Autodesk Inventor part; units mm, degrees
ref_plane "YZ Plane" through (0, 0, 0) normal (1, 0, 0) x (0, 1, 0)
ref_plane "XZ Plane" through (0, 0, 0) normal (0, 1, 0) x (-1, 0, 0)
ref_plane "XY Plane" through (0, 0, 0) normal (0, 0, 1) x (1, 0, 0)
sketch "Sketch1" plane through (0, 0, 0) normal (0, 1, 0) x (-1, 0, 0)
  line L0 (24.9723, 27.098) -> (-43.9316, 27.098)
  line L1 (-43.9316, 27.098) -> (-43.9316, -17.4091)
  line L2 (-43.9316, -17.4091) -> (24.9723, -17.4091)
  line L3 (24.9723, -17.4091) -> (24.9723, 27.098)
  circle A0 centre (9.5704, -1.5056) radius 3.81
  circle A1 centre (-3.1296, -1.5056) radius 3.81
  circle A2 centre (-15.8296, -1.5056) radius 3.81
  circle A3 centre (-28.5296, -1.5056) radius 3.81
  circle A4 centre (9.5704, 11.1944) radius 3.81
  circle A5 centre (-3.1296, 11.1944) radius 3.81
  circle A6 centre (-15.8296, 11.1944) radius 3.81
  circle A7 centre (-28.5296, 11.1944) radius 3.81
  line L4 (24.9723, -17.4091) -> (23.4483, -17.4091)
  line L5 (23.4483, -17.4091) -> (23.4483, 27.098)
  line L6 (-43.9316, -17.4091) -> (-42.4076, -17.4091)
  line L7 (-42.4076, -17.4091) -> (-42.4076, 27.098)
  point P0 (0, 0)
  dimension "d3" = 12.7
  dimension "d6" = 12.7
  dimension "d9" = 1.524
  dimension "d10" = 1.524
extrude "Extrusion1" add sketch "Sketch1" against normal blind 1.905 contours L5 L2 L7 L0 | A0 | A1 | A2 | A3 | A4 | A5 | A6 | A7
extrude "Extrusion2" add sketch "Sketch1" along normal blind 2.54 contours A0 | A1 | A2 | A3 | A4 | A5 | A6 | A7
chamfer "Chamfer1" distance 3.556 distance2 2.54 1 edges at (-5.7604, 2.54, 11.1944) measured on face at (-7.8424, 2.54, 10.6775)
chamfer "Chamfer2" distance 3.556 distance2 2.54 1 edges at (-5.7604, 2.54, -1.5056) measured on face at (-9.9176, 2.54, -0.5901)
chamfer "Chamfer3" distance 3.556 distance2 2.54 1 edges at (6.9396, 2.54, -1.5056) measured on face at (2.4763, 2.54, -0.5901)
chamfer "Chamfer4" distance 3.556 distance2 2.54 1 edges at (19.6396, 2.54, -1.5056) measured on face at (16.7802, 2.54, -2.3477)
chamfer "Chamfer5" distance 3.556 distance2 2.54 1 edges at (32.3396, 2.54, -1.5056) measured on face at (28.1824, 2.54, -0.5901)
chamfer "Chamfer6" distance 3.556 distance2 2.54 1 edges at (6.9396, 2.54, 11.1944) measured on face at (2.382, 2.54, 9.9337)
chamfer "Chamfer7" distance 3.556 distance2 2.54 1 edges at (19.6396, 2.54, 11.1944) measured on face at (16.7802, 2.54, 10.3523)
chamfer "Chamfer8" distance 3.556 distance2 2.54 1 edges at (32.3396, 2.54, 11.1944) measured on face at (28.1824, 2.54, 12.1099)
sketch "Sketch2" plane through (42.4076, 0, 27.098) normal (1, 0, 0) x (0, 0, -1)
  line L0 (19.1798, 6.2965) -> (19.1798, 7.6808)
  arc A0 (21.1991, 9.7001) -> (19.1798, 7.6808) centre (21.1991, 7.6808) ccw
  line L1 (21.1991, 9.7001) -> (26.1711, 9.7001)
  arc A1 (27.8729, 7.9983) -> (26.1711, 9.7001) centre (26.1711, 7.9983) ccw
  line L2 (27.8729, 7.9983) -> (27.8729, 6.2965)
  arc A2 (27.2379, 5.6615) -> (27.8729, 6.2965) centre (27.2379, 6.2965) ccw
  line L3 (27.2379, 5.6615) -> (19.8148, 5.6615)
  arc A3 (19.1798, 6.2965) -> (19.8148, 5.6615) centre (19.8148, 6.2965) ccw
  line L4 (26.8541, 21.209) -> (26.8541, 19.8247)
  arc A4 (24.8348, 17.8054) -> (26.8541, 19.8247) centre (24.8348, 19.8247) ccw
  line L5 (24.8348, 17.8054) -> (19.8628, 17.8054)
  arc A5 (18.161, 19.5072) -> (19.8628, 17.8054) centre (19.8628, 19.5072) ccw
  line L6 (18.161, 19.5072) -> (18.161, 21.209)
  arc A6 (18.796, 21.844) -> (18.161, 21.209) centre (18.796, 21.209) ccw
  line L7 (18.796, 21.844) -> (26.2191, 21.844)
  arc A7 (26.8541, 21.209) -> (26.2191, 21.844) centre (26.2191, 21.209) ccw
  line L8 (44.5071, 3.302) -> (0, 3.302)
  line L9 (44.5071, 3.302) -> (47.4281, 6.7381)
  line L10 (47.4281, 6.7381) -> (47.4281, 7.7839)
  line L11 (44.5071, 7.7839) -> (44.5071, 27.94)
  line L12 (42.6021, 27.94) -> (44.5071, 27.94)
  line L13 (42.6021, 26.9875) -> (42.6021, 27.94)
  line L14 (42.6021, 26.9875) -> (43.5546, 26.9875)
  line L15 (43.5546, 26.035) -> (43.5546, 26.9875)
  line L16 (0.9525, 26.035) -> (43.5546, 26.035)
  line L17 (0.9525, 26.035) -> (0.9525, 26.9875)
  line L18 (0.9525, 26.9875) -> (1.905, 26.9875)
  line L19 (1.905, 26.9875) -> (1.905, 27.94)
  line L20 (0, 27.94) -> (1.905, 27.94)
  line L21 (0, 7.7839) -> (0, 27.94)
  line L22 (0, 7.7839) -> (-2.921, 7.7839)
  line L23 (-2.921, 7.7839) -> (-2.921, 6.7381)
  line L24 (-2.921, 6.7381) -> (0, 3.302)
  line L25 (0, 0) -> (44.5071, 0)
  line L26 (0, -1.905) -> (-5.2131, 4.2274)
  line L27 (0, 3.302) -> (2.807, 0)
  line L28 (2.807, 0) -> (2.241, 0)
  line L29 (2.241, 0) -> (-3.429, 6.6699)
  line L30 (-2.921, 6.7381) -> (-3.429, 6.7381)
  line L31 (-3.429, 6.7381) -> (-3.429, 6.6699)
  line L32 (-3.429, 6.7381) -> (-3.429, 7.7839)
  line L33 (-3.429, 7.7839) -> (-3.429, 8.2919)
  line L34 (-2.921, 7.7839) -> (-1.651, 7.7839)
  line L35 (-1.651, 7.7839) -> (0, 5.8417)
  line L36 (-5.969, 8.2919) -> (-5.969, 5.6615)
  line L37 (-5.8869, 5.0201) -> (-5.969, 5.1167)
  line L38 (-5.969, 5.6615) -> (-5.969, 6.2838)
  line L39 (0, 6.2616) -> (-2.286, 8.9508)
  line L40 (-2.286, 8.9508) -> (-3.429, 7.9791)
  line L41 (-0.1085, 6.3892) -> (-0.1085, 8.8286)
  line L42 (-1.3785, 10.0986) -> (-2.794, 10.0986)
  line L43 (-5.969, 6.9236) -> (-5.969, 8.2919)
  arc A8 (-2.794, 10.0986) -> (-5.969, 6.9236) centre (-2.794, 6.9236) ccw
  line L44 (47.4281, 7.7839) -> (47.4281, 6.7381)
  line L45 (47.4281, 6.7381) -> (47.9361, 6.7381)
  line L46 (47.9361, 6.7381) -> (47.9361, 6.6699)
  line L47 (47.9361, 6.7381) -> (47.9361, 7.7839)
  line L48 (47.9361, 7.7839) -> (47.9361, 8.2919)
  line L49 (46.7931, 8.9508) -> (47.9361, 7.9791)
  arc A9 (50.4761, 6.9236) -> (47.3011, 10.0986) centre (47.3011, 6.9236) ccw
  line L50 (50.4761, 6.9236) -> (50.4761, 8.2919)
  line L51 (50.4761, 8.2919) -> (50.4761, 6.2838)
  line L52 (50.4761, 5.6615) -> (50.4761, 5.1167)
  line L53 (50.394, 5.0201) -> (50.4761, 5.1167)
  line L54 (47.4281, 6.7381) -> (44.5071, 3.302)
  line L55 (41.7002, 0) -> (42.2662, 0)
  line L56 (44.6156, 6.3892) -> (44.6156, 8.8286)
  line L57 (44.5071, 3.302) -> (41.7002, 0)
  line L58 (44.5071, 6.2616) -> (46.7931, 8.9508)
  line L59 (45.8856, 10.0986) -> (47.3011, 10.0986)
  line L60 (42.2662, 0) -> (47.9361, 6.6699)
  line L61 (44.5071, -1.905) -> (49.7202, 4.2274)
  line L62 (44.5071, 0) -> (44.5071, -1.905)
  line L63 (0, 0) -> (0, -1.905)
  line L64 (0, -1.905) -> (0, 0)
  line L65 (0, 0) -> (2.241, 0)
  line L66 (44.5071, -1.905) -> (44.5071, 0)
  line L67 (44.5071, 0) -> (42.2662, 0)
  arc A10 (-5.969, 6.2838) -> (-5.2131, 4.2274) centre (-2.794, 6.2838) ccw
  arc A11 (49.7202, 4.2274) -> (50.4761, 6.2838) centre (47.3011, 6.2838) ccw
  arc A12 (-0.1085, 8.8286) -> (-1.3785, 10.0986) centre (-1.3785, 8.8286) ccw
  arc A13 (45.8856, 10.0986) -> (44.6156, 8.8286) centre (45.8856, 8.8286) ccw
  point P0 (27.098, 0)
  point P1 (2.3019, 5.207)
  point P2 (-0.1085, 10.0986)
  point P3 (58.983, -0.9263)
  point P4 (58.983, -2.8313)
  point P5 (42.2053, 5.207)
  point P6 (44.6156, 10.0986)
  point P7 (50.4761, 6.9236)
  point P8 (-1.2941, 7.7839)
  point P9 (-0.1085, 7.7839)
  dimension "d41" = 3.302
  dimension "d42" = 0.508
  dimension "d43" = 0.508
  dimension "d44" = 1.27
  dimension "d45" = 2.54
  dimension "d46" = 3.175
  dimension "d53" = 3.175
  dimension "d56" = 1.27
extrude "Extrusion3" add sketch "Sketch2" against normal up to surface (65.8559 mm away) contours L47 L48 L49 L58 L56 A13 L59 A9 L51 A11 L61 L62 L25 L60 L46 | L31 L29 L25 L63 L26 A10 L36 A8 L42 A12 L41 L22 L39 L40 L33 L32 | L22 L41 L39
properties part number "ControllerClamp"
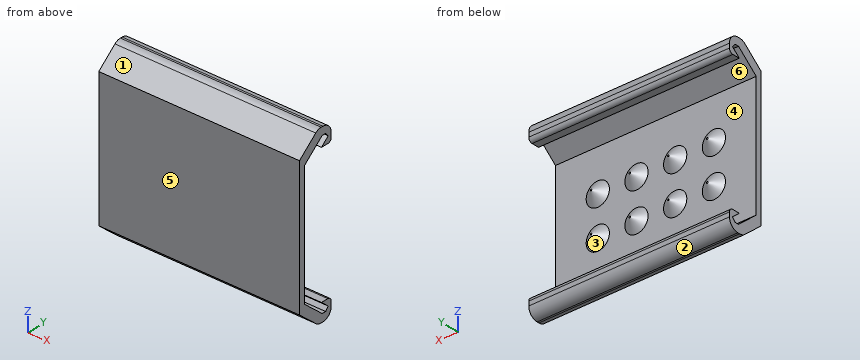
Could you check a few things on this model? Use its own coordinates, in mm. Face numbers are marked on the shaded views. A direction names the side the tool comes from. Round coordinates to 2 decimals unless told otherwise and drop trailing zeros. Order: outer loops, then holes, each group sorted by start corner. A loop starts at its lowest first (then second) coordinate and runs counter-clockwise, first axis right, second up.
(1) Please list where these lines run through material, in increasing order: line 1 along X through (y, z) = (2, -2); line 2 along Y through (x, z) = (32, 6) (3 decimals); line 3 along X through (y, z) = (0.25, 10).
Response values:
line 1: x = -10.45 to -8.69, 2.25 to 4.01, 14.95 to 16.71, 27.65 to 29.41
line 2: y = -1.905 to 0
line 3: x = -12.82 to -6.32, -0.12 to 6.38, 12.58 to 19.08, 25.28 to 31.78
(2) Imagine slicing it at D-D (y = -1). Write out the boundary of the cut face in (x, z), plus the area to 3 significant figures.
Response values:
outline: (-23.45, -18.18) - (42.41, -18.18) - (42.41, 27.87) - (-23.45, 27.87) - close
area: 3,030 mm2
(3) Imagine slicing it at A-A (y = 5). Write out the boundary of the cut face in (x, z), plus the area to 3 significant figures.
Response values:
outline: (-23.45, -23.11) - (42.41, -23.11) - (42.41, -19.42) - (-23.45, -19.42) - close; (-23.45, 29.11) - (42.41, 29.11) - (42.41, 32.8) - (-23.45, 32.8) - close
area: 486 mm2
(4) Which directions (+Z, -Z, +X, -X, +Y, -Y) give clear straight access to the entire face, cutting with the end or side of a thin tool? Please do the marked faces 4, 5 and 6.
Response values:
face 4: +Y
face 5: +Z, -Z, +X, -X, -Y
face 6: +X, -X
(5) I'm going to push flat-ended pins straight in: pin 1 (5 mm diameter, centred on x = -3.5, z = -9, fed in from +Y); pin 2 (1 mm diameter, centred on x = 16, y = 0, fed in from +Z); pin 3 (5 mm diameter, centred on x = -10.5, y = 2.5, fed in from -Z). Where does each tip first touch, or does it pass through?
Response values:
pin 1: stops at y = 0
pin 2: stops at z = 29.14
pin 3: stops at z = -23.11
(6) Imagine slicing it at C-C (z = -9). Write out the boundary of the cut face in (x, y) (3 decimals), plus the area to 3 significant figures.
Response values:
outline: (-23.448, -1.905) - (42.408, -1.905) - (42.408, 0) - (-23.448, 0) - close
area: 125 mm2
(7) If we mould it in two halves opening along Z, with no side actions, what happens to the marked faces 1, 2 and 3? For each: released by +Z, released by -Z, zero draft, split by the parting line, or undercut.
Response values:
face 1: released by +Z
face 2: released by -Z
face 3: undercut
